Autodesk Fusion 360 part; units mm, degrees
sketch "スケッチ1" plane through (0, 0, 0) normal (0, 0, 1) x (1, 0, 0)
  line L0 (-3.5, 31.5) -> (3.5, 31.5)
  line L1 (3.5, 31.5) -> (17.5, 17.5)
  line L2 (17.5, 17.5) -> (17.5, -17.5)
  line L3 (17.5, -17.5) -> (3.5, -31.5)
  line L4 (3.5, -31.5) -> (-3.5, -31.5)
  line L5 (-3.5, -31.5) -> (-17.5, -17.5)
  line L6 (-17.5, -17.5) -> (-17.5, 17.5)
  line L7 (-17.5, 17.5) -> (-3.5, 31.5)
  circle A0 centre (-12.5, 12.5) radius 3
  circle A1 centre (-12.5, -12.5) radius 3
  circle A2 centre (12.5, -12.5) radius 3
  circle A3 centre (12.5, 12.5) radius 3
  dimension "d1" = 35
  dimension "d2" = 63
  dimension "d3" = 31.5
  dimension "d4" = 17.5
  dimension "d5" = 14
  dimension "d6" = 14
  dimension "d7" = 14
  dimension "d8" = 14
  dimension "d9" = 14
  dimension "d10" = 14
  dimension "d11" = 14
  dimension "d12" = 14
  dimension "d13" = 6
  dimension "d14" = 12.5
  dimension "d15" = 12.5
  dimension "d17" = 360
extrude "押し出し1" add sketch "スケッチ1" along normal blind 12.5 contours L0 L1 L2 L3 L4 L5 L6 L7 | A0 | A1 | A2 | A3
extrude "押し出し2" cut sketch "スケッチ1" along normal blind 3 contours A0 | A1 | A2 | A3
sketch "スケッチ2" plane through (17.5, 0, 0) normal (1, 0, 0) x (0, 1, 0)
  line L0 (-17.5, 0) -> (17.5, 0)
  line L1 (17.5, 0) -> (17.5, 12.5)
  line L2 (17.5, 12.5) -> (-17.5, 12.5)
  line L3 (-17.5, 12.5) -> (-17.5, 0)
  circle A0 centre (0, 12.75) radius 9.5
  line L4 (17.5, 0) -> (-17.5, 0)
  dimension "d22" = 19
  dimension "d23" = 12.75
extrude "押し出し3" cut sketch "スケッチ2" against normal up to surface (35 mm away) contours L2 A0 picked at (1.5592, 9.8271)
sketch "スケッチ3" plane through (0, 0, 12.5) normal (0, 0, 1) x (-1, 0, 0)
  line L0 (17.5, -9.4967) -> (-17.5, -9.4967)
  line L1 (-17.5, -9.4967) -> (-17.5, -17.5)
  line L2 (-17.5, -17.5) -> (-3.5, -31.5)
  line L3 (-3.5, -31.5) -> (3.5, -31.5)
  line L4 (3.5, -31.5) -> (17.5, -17.5)
  line L5 (17.5, -17.5) -> (17.5, -9.4967)
  circle A0 centre (12.5, -12.5) radius 1.75
  circle A1 centre (12.5, 12.5) radius 1.75
  circle A2 centre (-12.5, 12.5) radius 1.75
  circle A3 centre (-12.5, -12.5) radius 1.75
  line L6 (-3.5, 31.5) -> (3.5, 31.5)
  line L7 (0, 31.5) -> (0, -31.5) construction
  circle A4 centre (0, 22.5) radius 5.5
  circle A5 centre (0, -22.5) radius 5.5
  point P0 (12.5, -12.5)
  dimension "d26" = 3.5
  dimension "d28" = 360
  dimension "d32" = 11
  dimension "d33" = 11
  dimension "d34" = 9
  dimension "d35" = 9
extrude "押し出し4" cut sketch "スケッチ3" against normal blind 9.1 contours A0 | A1 | A2 | A3
extrude "押し出し5" cut sketch "スケッチ3" against normal through all contours A4 | A5
fillet "フィレット1" radius 5 8 edges at (-17.5, 17.5, 6.25) (-3.5, 31.5, 6.25) (3.5, 31.5, 6.25) (17.5, 17.5, 6.25) (-17.5, -17.5, 6.25) (-3.5, -31.5, 6.25) (3.5, -31.5, 6.25) (17.5, -17.5, 6.25)
equation "d3 = d2 / 2"
equation "d4 = d1 / 2"
equation "d7 = d5"
equation "d8 = d6"
equation "d9 = d5"
equation "d10 = d7"
equation "d11 = d10"
equation "d12 = d9"
Geometry check sheet. Reference: the model listing, model coordinates, mm. A direction names the side the tool comes from. Round coordinates to 2 decimals unless told otherwise and drop trailing zeros. Loops run counter-clockwise (first coordinate to the right, second up) from the corner with the lowest first, then second, coordinate; pieces in that order, holes last. Notation, with made-up numbers: (-19.75, -11) - (33.25, -11) arc R25 ccw to (33.25, 19) - close; hole circle Ø4 at (65, 82). An arc over 180 degrees is marked (long way). Answer as CSV lines item,"result".
(1) Cross-section at B-B, the plane y = 22.5. Enter the section's corners in (x, z).
Output values:
outline,"(-12.5, 0) - (-5.5, 0) - (-5.5, 12.5) - (-12.5, 12.5) - close; (5.5, 0) - (12.5, 0) - (12.5, 12.5) - (5.5, 12.5) - close"
(2) Cross-section at C-C, the plane z = 8. Enter the section's corners in (x, y), and give its area (3 significant figures).
Output values:
outline,"(-17.5, -15.43) arc R5 ccw to (-16.04, -18.96) - (-4.96, -30.04) arc R5 ccw to (-1.43, -31.5) - (1.43, -31.5) arc R5 ccw to (4.96, -30.04) - (16.04, -18.96) arc R5 ccw to (17.5, -15.43) - (17.5, -8.23) - (-17.5, -8.23) - close; (-17.5, 8.23) - (17.5, 8.23) - (17.5, 15.43) arc R5 ccw to (16.04, 18.96) - (4.96, 30.04) arc R5 ccw to (1.43, 31.5) - (-1.43, 31.5) arc R5 ccw to (-4.96, 30.04) - (-16.04, 18.96) arc R5 ccw to (-17.5, 15.43) - close; hole circle Ø3.5 at (-12.5, -12.5); hole circle Ø3.5 at (-12.5, 12.5); hole circle Ø11 at (0, -22.5); hole circle Ø11 at (0, 22.5); hole circle Ø3.5 at (12.5, -12.5); hole circle Ø3.5 at (12.5, 12.5)"
area,"1,000 mm²"
(3) Set-up check for faces 4 (the face through (-14.9, 14.3, 1.5)), 5 (the face through (13, 12, 3.4)), 6 (the face through (0.716, -27.953, 6.338)): record each of +Z, -Z, +X, -X, +Y, -Y from which the full face is reachable in a straight line by a thin tool's end or side.
Output values:
face 4,"-Z"
face 5,"+Z"
face 6,"+Z, -Z"
(4) Depth check by flat-ended pin: pin 1 Ø5.5 at (x, y) = (-12.5, 12.5) entering from -Z; pin 2 Ø1.8 at (x, y) = (13, -12.5) entering from +Z; pin 3 Ø6 at (y, z) = (24, 7) entering from -X. Enter the tip coordinate at first touch or a pass-through.
Output values:
pin 1,"stops at z = 3"
pin 2,"stops at z = 3.4"
pin 3,"stops at x = -14"
(5) Material ranges on line 1 along X through (y, z) = (-12.5, 8.25); line 2 along Y through (x, z) = (-12.5, 12); line 3 along Y through (x, z) = (-12.5, 2), recorded low to high.
Output values:
line 1,"x = -17.5 to -14.25, -10.75 to 10.75, 14.25 to 17.5"
line 2,"y = -22.5 to -14.25, -10.75 to -9.47, 9.47 to 10.75, 14.25 to 22.5"
line 3,"y = -22.5 to -15.5, -9.5 to 9.5, 15.5 to 22.5"
(6) Cross-section at D-D, the plane y = 12.5. Enter the section's corners in (x, z).
Output values:
outline,"(-17.5, 0) - (-15.5, 0) - (-15.5, 3) - (-9.5, 3) - (-9.5, 0) - (9.5, 0) - (9.5, 3) - (15.5, 3) - (15.5, 0) - (17.5, 0) - (17.5, 12.5) - (14.25, 12.5) - (14.25, 3.4) - (10.75, 3.4) - (10.75, 12.5) - (-10.75, 12.5) - (-10.75, 3.4) - (-14.25, 3.4) - (-14.25, 12.5) - (-17.5, 12.5) - close"
(7) Release check for a two-part mould opening along Y. For faces 1 (the face through (17.13, 17.32, 6.34)), 2 (the face through (-12, 12, 3.4)), 3 (the face through (-3.37, -31.11, 6.34)) record: released by +Y, released by -Y, zero draft, split by the parting line, or undercut.
Output values:
face 1,"released by +Y"
face 2,"undercut"
face 3,"released by -Y"
